Verification items for this drawing (mm, ordinates from the low corner). Round coordinates to 2 decimals unless told otherwise and drop trailing zeros. Order: outer loops, then holes, each group sorted by start corner. A loop starts at its lowest first (then second) coordinate and runs counter-clockwise, first axis right, second up. Notation, with made-up numbers: (-28, 58.5) - (-9, 58.5) arc R35 ccw to (-9, 93.5) - close; hole circle Ø6 at (26.5, -0.75). An arc over 180 degrees is marked (long way). Use a Markdown table: item, result. Add a question column.
(1) Section check A-A on y = 36. Record the boundary of the cut face in (x, z) (1 decimal), then the cut area to 4 significant figures.
(2) Mould release check, pull along Y, two halves, no side actions. Record for the marked faces 1 and 2: released by +Y, released by -Y, zero draft, split by the parting line, or undercut.
(3) Gauge pin test, flat ends, axial feed: P1, Ø3, axis at x = 156, y = 47.5, coming from the +Z side; P2, Ø5, axis at y = 76.5, z = 86.5, coming from the -X side; P3, Ø2, axis at y = 19, z = 75, coming from the +X side; P4, Ø14.5, axis at y = 48, z = 61, coming from the +X side. Record the tip position at first contact, or that the pin passes through.
(4) Section check C-C on x = 123.5. Record the boundary of the cut face in (y, z) (1 decimal).
(5) Section check B-B on z = 16.5. Record the boundary of the cut face in (x, y), then the cut area to 3 significant figures.
(6) Section check D-D on z = 41. Record the boundary of the cut face in (x, y) (1 decimal), then the cut area to 3 significant figures.
(7) Thickness scan on line 1 along X through (y, z) = (76, 29); line 2 along X through (y, z) = (74.5, 61) (1 decimal); line 3 along Z through (x, y) = (118.5, 16) (1 decimal). Record the ranges inside material, lowest first. Write a range as [from, to].
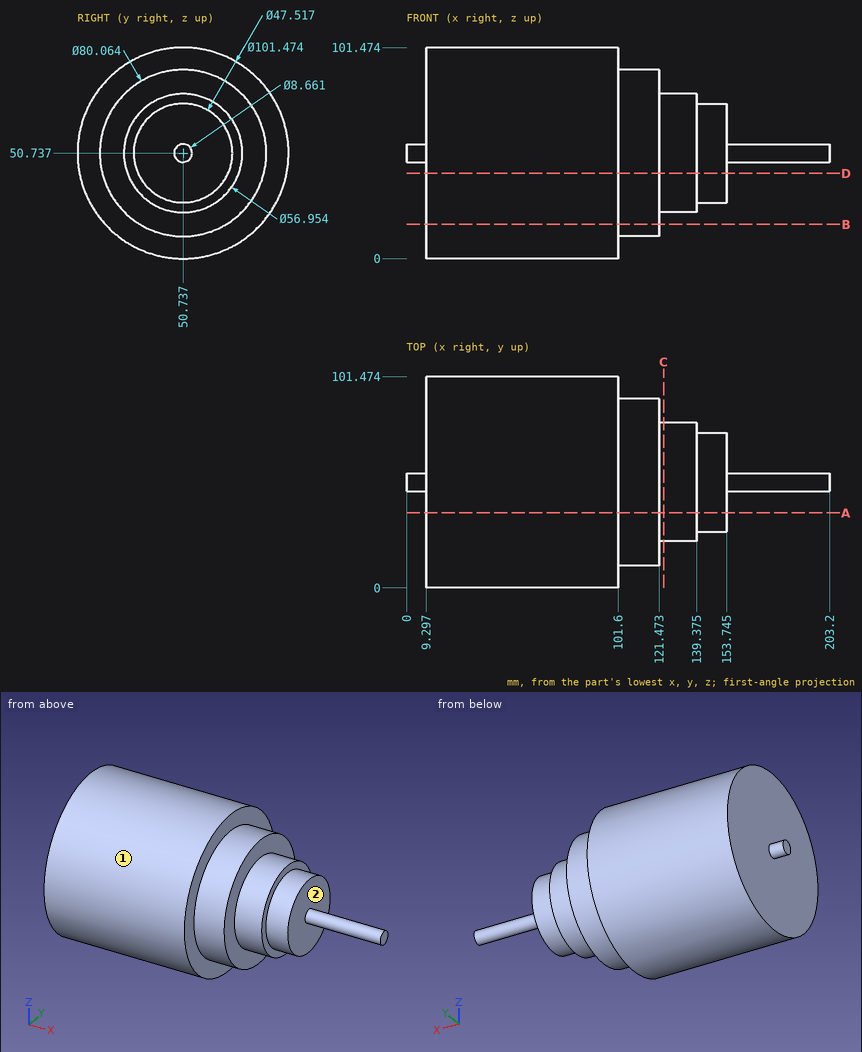
Check sheet entries:
| question | item | result |
|---|---|---|
| 1 | outline | (9.3, 2.2) - (101.6, 2.2) - (101.6, 13.5) - (121.5, 13.5) - (121.5, 26.4) - (139.4, 26.4) - (139.4, 32.1) - (153.7, 32.1) - (153.7, 69.4) - (139.4, 69.4) - (139.4, 75.1) - (121.5, 75.1) - (121.5, 88) - (101.6, 88) - (101.6, 99.3) - (9.3, 99.3) - close |
| 1 | area | 11,850 mm2 |
| 2 | face 1 | split by the parting line |
| 2 | face 2 | zero draft |
| 3 | P1 | stops at z = 54.7 |
| 3 | P2 | stops at x = 9.3 |
| 3 | P3 | stops at x = 121.47 |
| 3 | P4 | stops at x = 203.2 |
| 4 | outline | circle Ø57 at (50.7, 50.7) |
| 5 | outline | (9.3, 13.29) - (101.6, 13.29) - (101.6, 29.99) - (121.47, 29.99) - (121.47, 71.48) - (101.6, 71.48) - (101.6, 88.18) - (9.3, 88.18) - close |
| 5 | area | 7,740 mm2 |
| 6 | outline | (9.3, 0.9) - (101.6, 0.9) - (101.6, 11.9) - (121.5, 11.9) - (121.5, 24) - (139.4, 24) - (139.4, 29.1) - (153.7, 29.1) - (153.7, 72.4) - (139.4, 72.4) - (139.4, 77.5) - (121.5, 77.5) - (121.5, 89.6) - (101.6, 89.6) - (101.6, 100.5) - (9.3, 100.5) - close |
| 6 | area | 12,300 mm2 |
| 7 | line 1 | x = [9.3, 121.47] |
| 7 | line 2 | x = [9.3, 139.4] |
| 7 | line 3 | z = [30.8, 70.6] |
